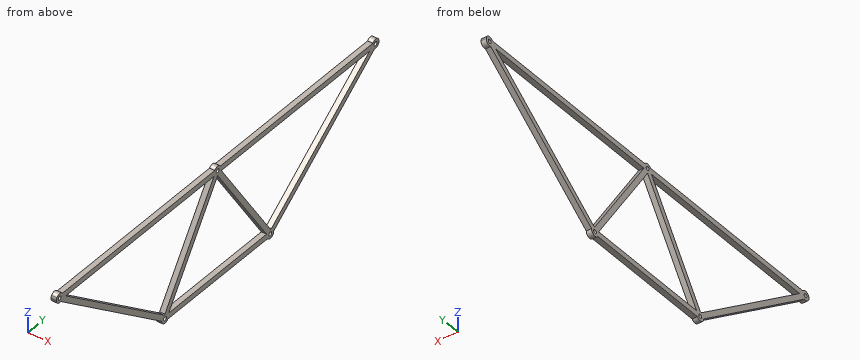
```python
from build123d import *

# Parameters (mm, degrees)
BOSS_EXTRUDE1_DEPTH = 15
SKETCH3_R           = 13
BOSS_EXTRUDE2_DEPTH = 15
CUT_EXTRUDE1_DEPTH  = 15
SKETCH5_R           = 5.5
CUT_EXTRUDE2_DEPTH  = 15


with BuildPart() as part:
    # Sketch2 → Boss-Extrude1 (new body)
    with BuildSketch(Plane.YZ):
        with BuildLine():
            Line((600, 307.5), (-22.5, 307.5))
            Line((-22.5, 307.5), (395.5, -6))
            ThreePointArc((395.5, -6), (397.628291755, -7.115124735), (400, -7.5))
            Line((400, -7.5), (800, -7.5))
            ThreePointArc((800, -7.5), (802.371708245, -7.115124735), (804.5, -6))
            Line((804.5, -6), (1222.5, 307.5))
            Line((1222.5, 307.5), (600, 307.5))
        make_face()
        Polygon((414.013878189, 7.5), (600, 286.479182717), (785.986121811, 7.5), align=None, mode=Mode.SUBTRACT)
        Polygon((801.842585459, 10.756939094), (614.013878189, 292.5), (1177.5, 292.5), align=None, mode=Mode.SUBTRACT)
        Polygon((585.986121811, 292.5), (22.5, 292.5), (398.157414541, 10.756939094), align=None, mode=Mode.SUBTRACT)
    extrude(amount=BOSS_EXTRUDE1_DEPTH)

    # Sketch3 → Boss-Extrude2 (add)
    with BuildSketch(Plane.YZ.offset(15)):
        with Locations((400, 0)):
            Circle(SKETCH3_R)
        with Locations((0, 300)):
            Circle(SKETCH3_R)
        with Locations((600, 300)):
            Circle(SKETCH3_R)
        with Locations((1200, 300)):
            Circle(SKETCH3_R)
        with Locations((800, 0)):
            Circle(SKETCH3_R)
    extrude(amount=-BOSS_EXTRUDE2_DEPTH)

    # Sketch4 → Cut-Extrude1 (cut)
    with BuildSketch(Plane.YZ.offset(15)):
        with BuildLine():
            Line((-10.618380291, 307.5), (-22.5, 307.5))
            Line((-22.5, 307.5), (-12.994704233, 300.371028174))
            ThreePointArc((-12.994704233, 300.371028174), (-12.332882875, 304.110960958), (-10.618380291, 307.5))
        make_face()
        with BuildLine():
            Line((1210.618380291, 307.5), (1222.5, 307.5))
            Line((1222.5, 307.5), (1212.994704233, 300.371028174))
            ThreePointArc((1212.994704233, 300.371028174), (1212.332882875, 304.110960958), (1210.618380291, 307.5))
        make_face()
    extrude(amount=-CUT_EXTRUDE1_DEPTH, mode=Mode.SUBTRACT)

    # Sketch5 → Cut-Extrude2 (cut)
    with BuildSketch(Plane.YZ.offset(15)):
        with Locations(Location((0, 300, 0), (0, 0, 270))):
            Circle(SKETCH5_R)
        with Locations(Location((600, 300, 0), (0, 0, 270))):
            Circle(SKETCH5_R)
        with Locations(Location((1200, 300, 0), (0, 0, 270))):
            Circle(SKETCH5_R)
        with Locations(Location((800, 0, 0), (0, 0, 270))):
            Circle(SKETCH5_R)
        with Locations(Location((400, 0, 0), (0, 0, 270))):
            Circle(SKETCH5_R)
    extrude(amount=-CUT_EXTRUDE2_DEPTH, mode=Mode.SUBTRACT)


solid = part.part
```
Work out the finished part from the listing and answer in its coordinate system (mm). Round coordinates to 2 decimals unless told otherwise and drop trailing zeros. Write each loop counter-clockwise with the first axis right and the second up, starting at its lowest first coordinate (ties: lowest second). Pieces come first, ordered by that corner, then holes. Notation, with made-up numbers: (76, 75.5) - (124, 75.5) arc R10 cw to (124, 93.5) - close; hole circle Ø5 at (28.25, -32.75). An arc over 180 degrees is marked (long way). Return JSON: item names as keys, results as strings. Group by question number.
Q1. The part is cut by section B-B on y = 703.5. Write down the section's boundary in (x, z).
Q2. Find the intervals of material crossed by L1, parallel to Y at x = 4.5, z = 300; L2, parallel to Y at x = 10, z = 0; L3, parallel to Z at x = 8, y = 400, in increasing order.
Q3. The part is cut by section C-C on z = 163.5. Write down the section's boundary in (x, y).
Q4. The part is cut by section A-A on x = 4. Count the separate pieces of the cut face and the enclosed holes in it, then the cut area to 3 significant figures.
Q5. Each of these flat-tipped pins is pushed along its axis until it touches: pin 1 Ø6.5 at (y, z) = (0, 300) entering from +X; pin 2 Ø2 at (x, y) = (12, 340) entering from -Z (3 decimals); pin 3 Ø5 at (x, y) = (8, 363.5) entering from -Z (3 decimals); pin 4 Ø7.5 at (x, y) = (9, 970) entering from -Z. Where does it stop, or does it pass through?
Solved:
{
 "1": {"outline": "(0, -7.5) - (15, -7.5) - (15, 7.5) - (0, 7.5) - close; (0, 131.23) - (15, 131.23) - (15, 158.27) - (0, 158.27) - close; (0, 292.5) - (15, 292.5) - (15, 307.5) - (0, 307.5) - close"},
 "2": {"L1": "-13 to -5.5, 5.5 to 594.5, 605.5 to 1194.5, 1205.5 to 1213", "L2": "387 to 394.5, 405.5 to 794.5, 805.5 to 813", "L3": "-13 to -5.5, 5.5 to 13.52, 292.5 to 307.5"},
 "3": {"outline": "(0, 169.5) - (15, 169.5) - (15, 194.5) - (0, 194.5) - close; (0, 499.99) - (15, 499.99) - (15, 518.01) - (0, 518.01) - close; (0, 681.99) - (15, 681.99) - (15, 700.01) - (0, 700.01) - close; (0, 1005.5) - (15, 1005.5) - (15, 1030.5) - (0, 1030.5) - close"},
 "4": {"separate pieces": "1", "enclosed holes": "8", "area": "49,300 mm²"},
 "5": {"pin 1": "through", "pin 2": "z = 34.875", "pin 3": "z = 16.125", "pin 4": "z = 115.31"}
}
